Geometry: see drawing. Coordinates: mm, zero at the bounding-box minimum. A direction names the side the tool comes from. Give positions to 0.01 mm unless a question says otherwise; leave off trailing zeros. Write each loop counter-clockwise with the first axis right and the second up, starting at its lowest first coordinate (ties: lowest second). Pieces come first, ordered by that corner, then holes. Notation, with made-up numbers: M 19,-18.5 L 50,-18.5 A11 ccw 50,1.5 Z; hole C -22,-8 d8. An arc over 180 degrees is marked long. Use a Markdown table: item, result. Add a question column.
(1) Cut plane B-B (y = 6). Output: boundary loops of the cut face in (x, z) (1 decimal).
(2) Material intervals for L1, parallel to Z at x = 3.5, y = 1.75; L2, parallel to Y at x = 5.25, z = 6.25 (1 decimal); L3, parallel to X at y = 7.75, z = 10.5 (1 decimal), sorted ascending.
(3) Pin query (flat end, axial travel): pin 1 Ø1.5 at (x, z) = (5, 7) entering from -Y; pin 2 Ø1 at (x, z) = (8, 10) entering from -Y (1 decimal). Return the tip coordinate at first contact, or that it passes through.
(4) Cut plane C-C (z = 14). Output: boundary loops of the cut face in (x, y) (1 decimal).
(5) Reachability of the marked faces 1 and 2 from +Z, -Z, +X, -X, +Y, -Y: full face, straight path, thin tool, end or side. Return the list, or none.
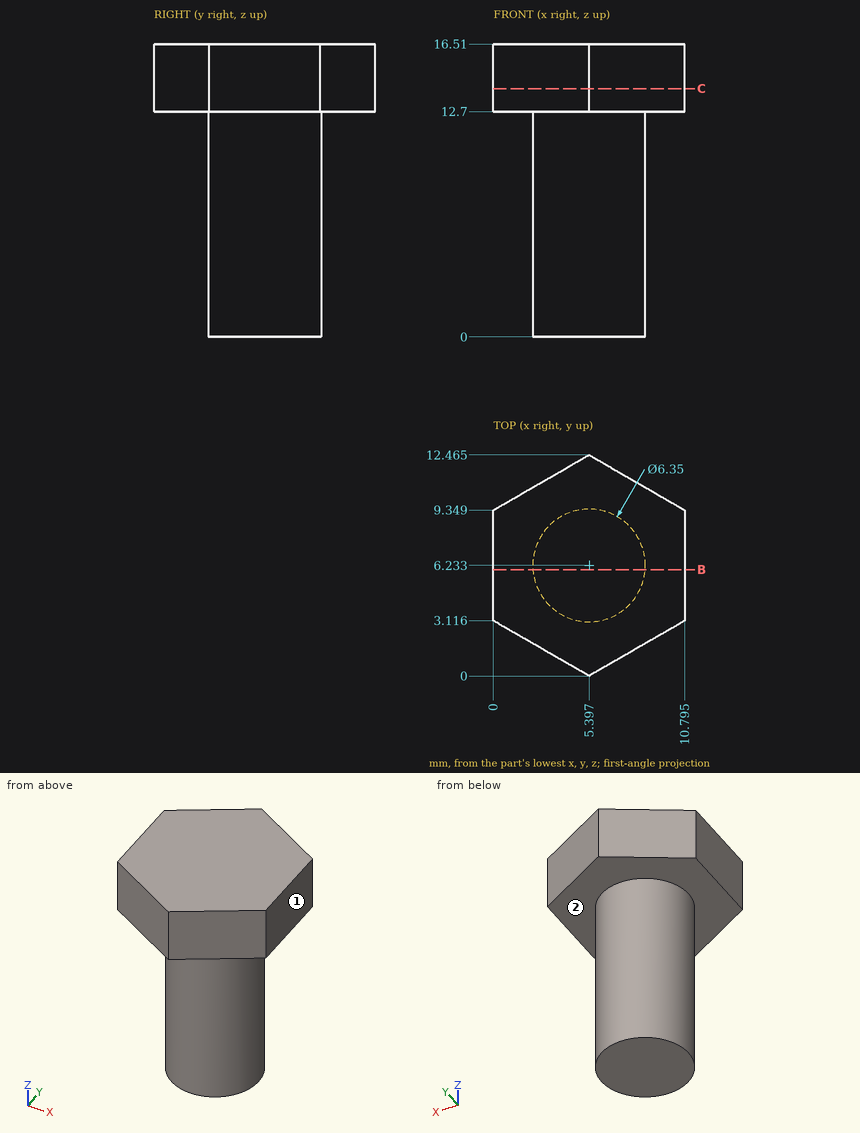
Answer list:
| question | item | result |
|---|---|---|
| 1 | outline | M 0,12.7 L 2.2,12.7 L 2.2,0 L 8.6,0 L 8.6,12.7 L 10.8,12.7 L 10.8,16.5 L 0,16.5 Z |
| 2 | L1 | 12.7 to 16.51 |
| 2 | L2 | 3.1 to 9.4 |
| 2 | L3 | 2.6 to 8.2 |
| 3 | pin 1 | y = 3.06 |
| 3 | pin 2 | y = 3.9 |
| 4 | outline | M 0,3.1 L 5.4,0 L 10.8,3.1 L 10.8,9.3 L 5.4,12.5 L 0,9.3 Z |
| 5 | face 1 | +Z, -Z, +X, +Y, -Y |
| 5 | face 2 | -Z |
